Input: part model. Units: mm. Frame: model coordinates. Face numbers are marked on the shaded views. A direction names the side the tool comes from. Coordinates: 2 decimals unless noted, no trailing zeros. Loops run counter-clockwise (first coordinate to the right, second up) from the corner with the lowest first, then second, coordinate; pieces in that order, holes last. Notation, with made-up numbers: M 39,4.25 L 82,4.25 A19 ccw 82,37.25 Z; hole C -1.75,-19.75 d11. An arc over 180 degrees is marked long. Use a Markdown table: item, result. Add a question column.
1. Pin query (flat end, axial travel): pin 1 (1.5 mm diameter, centred on x = 9.5, y = 1, fed in from +Z); pin 2 (1.5 mm diameter, centred on y = 1.5, z = -8.5, fed in from +X); pin 3 (3 mm diameter, centred on x = 10, z = -16, fed in from -Y). Return the tip coordinate at first contact, or that it passes through.
2. Draft query along Z for the marked faces 6, 7 and 8. Return one class per face: +Z half, -Z half, draft (parallel to the pull), parting line (faces both ways), or undercut.
3. Section B-B on z = -1.75. Output: boundary loops of the cut face in (x, y), then the cut area to 3 significant figures.
4. Line query: L1, parallel to Z at x = 10, y = 1; L2, parallel to X at y = 1.95, z = -11; L3, parallel to X at y = 1.5, z = -16. Output: solid intervals per line, ascending. Write a range as [from, to].
5. Section D-D on x = 12.25. Output: boundary loops of the cut face in (y, z), then the cut area to 3 significant figures.
6. Section A-A on y = 0.8. Output: boundary loops of the cut face in (x, z), then the cut area to 3 significant figures.
7. Set-up query: the marked faces 1, 2, 3, 4 and 5. Return all of +Z, -Z, +X, -X, +Y, -Y with unobstructed straight access to the full face (end or side cutting, diameter ignored); none if empty.
8. Section C-C on x = 10. Output: boundary loops of the cut face in (y, z), then the cut area to 3 significant figures.
```python
from build123d import *

# Parameters (mm, degrees)
SKETCH1_W               = 20
SKETCH1_H               = 20
BOSS_EXTRUDE1_DEPTH     = 3
SKETCH2_W               = 2.5
SKETCH2_H               = 12
CUT_EXTRUDE1_DEPTH      = 3
SKETCH3_R               = 1.6
CUT_EXTRUDE2_DEPTH      = 1
CUT_EXTRUDE2_DEPTH_BACK = 4
SKETCH4_W               = 5
SKETCH4_H               = 12
CUT_EXTRUDE3_DEPTH      = 1
CUT_EXTRUDE3_DEPTH_BACK = 4


with BuildPart() as part:
    # Sketch1 → Boss-Extrude1 (new body)
    with BuildSketch(Plane(origin=(0, 0, 0), x_dir=(1, 0, 0), z_dir=(0, 1, 0))):
        with Locations((10, 10)):
            Rectangle(SKETCH1_W, SKETCH1_H)
    extrude(amount=BOSS_EXTRUDE1_DEPTH)

    # Sketch2 → Cut-Extrude1 (cut)
    with BuildSketch(Plane(origin=(0, 3, 0), x_dir=(1, 0, 0), z_dir=(0, 1, 0))):
        with Locations((1.25, 6)):
            Rectangle(SKETCH2_W, SKETCH2_H)
    cut_extrude1 = extrude(amount=-CUT_EXTRUDE1_DEPTH, mode=Mode.SUBTRACT)

    # Mirror1: Cut-Extrude1 across plane
    add(cut_extrude1.mirror(Plane.ZY.offset(-10)), mode=Mode.SUBTRACT)

    # Sketch3 → Cut-Extrude2 (cut, two sides)
    with BuildSketch(Plane(origin=(0, 3, 0), x_dir=(1, 0, 0), z_dir=(0, 1, 0))) as cut_extrude2_sk:
        with Locations((10, 16)):
            Circle(SKETCH3_R)
    extrude(amount=CUT_EXTRUDE2_DEPTH, mode=Mode.SUBTRACT)
    extrude(cut_extrude2_sk.sketch, amount=-CUT_EXTRUDE2_DEPTH_BACK, mode=Mode.SUBTRACT)

    # Sketch4 → Cut-Extrude3 (cut, two sides)
    with BuildSketch(Plane(origin=(0, 3, 0), x_dir=(1, 0, 0), z_dir=(0, 1, 0))) as cut_extrude3_sk:
        with Locations((10, 6)):
            Rectangle(SKETCH4_W, SKETCH4_H)
    extrude(amount=CUT_EXTRUDE3_DEPTH, mode=Mode.SUBTRACT)
    extrude(cut_extrude3_sk.sketch, amount=-CUT_EXTRUDE3_DEPTH_BACK, mode=Mode.SUBTRACT)


solid = part.part
```
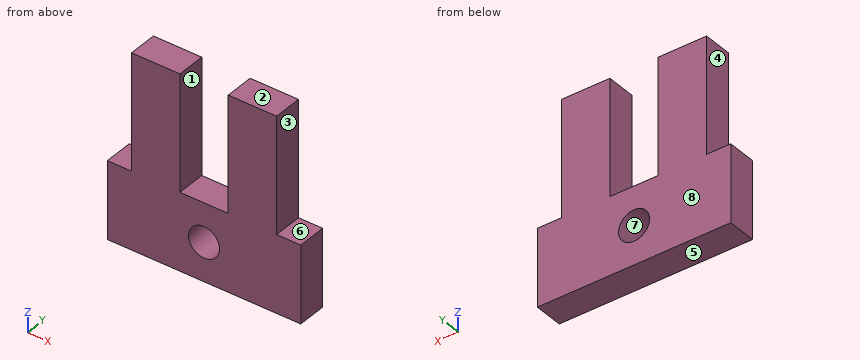
Answers below:
| question | item | result |
|---|---|---|
| 1 | pin 1 | stops at z = -12 |
| 1 | pin 2 | stops at x = 17.5 |
| 1 | pin 3 | passes through |
| 2 | face 6 | +Z half |
| 2 | face 7 | undercut |
| 2 | face 8 | draft |
| 3 | outline | M 2.5,0 L 7.5,0 L 7.5,3 L 2.5,3 Z; M 12.5,0 L 17.5,0 L 17.5,3 L 12.5,3 Z |
| 3 | area | 30.0 mm² |
| 4 | L1 | z = [-20, -17.6], [-14.4, -12] |
| 4 | L2 | x = [2.5, 7.5], [12.5, 17.5] |
| 4 | L3 | x = [0, 8.4], [11.6, 20] |
| 5 | outline | M 0,-20 L 3,-20 L 3,-12 L 0,-12 Z |
| 5 | area | 24.0 mm² |
| 6 | outline | M 0,-20 L 20,-20 L 20,-12 L 17.5,-12 L 17.5,0 L 12.5,0 L 12.5,-12 L 7.5,-12 L 7.5,0 L 2.5,0 L 2.5,-12 L 0,-12 Z; hole C 10,-16 d3.2 |
| 6 | area | 272 mm² |
| 7 | face 1 | +Z, +Y, -Y |
| 7 | face 2 | +Z, +X, -X, +Y, -Y |
| 7 | face 3 | +Z, +X, +Y, -Y |
| 7 | face 4 | +Z, -X, +Y, -Y |
| 7 | face 5 | -Z, +X, -X, +Y, -Y |
| 8 | outline | M 0,-20 L 3,-20 L 3,-17.6 L 0,-17.6 Z; M 0,-14.4 L 3,-14.4 L 3,-12 L 0,-12 Z |
| 8 | area | 14.4 mm² |
